Autodesk Inventor part; units mm, degrees
ref_plane "YZ Plane" through (0, 0, 0) normal (1, 0, 0) x (0, 1, 0)
ref_plane "XZ Plane" through (0, 0, 0) normal (0, 1, 0) x (-1, 0, 0)
ref_plane "XY Plane" through (0, 0, 0) normal (0, 0, 1) x (1, 0, 0)
sketch "スケッチ1" plane through (0, 0, 0) normal (0, 0, 1) x (1, 0, 0)
  line L0 (195, -7.5) -> (-195, -7.5)
  line L1 (-195, -7.5) -> (-195, 7.5)
  line L2 (-195, 7.5) -> (195, 7.5)
  line L3 (195, 7.5) -> (195, -7.5)
  line L4 (195, -7.5) -> (-195, 7.5) construction
  line L5 (-195, -7.5) -> (195, 7.5) construction
  circle A0 centre (0, 70.8153) radius 120
  line L6 (0, -7.5) -> (0, 7.5)
  circle A1 centre (-127.5, -22.5) radius 38
  line L7 (-175, -5) -> (-145, -5)
  line L8 (-145, -5) -> (-145, 5)
  line L9 (-145, 5) -> (-175, 5)
  line L10 (-175, 5) -> (-175, -5)
  line L11 (-195, 0) -> (195, 0)
  circle A2 centre (-175, 0) radius 1.6
  circle A3 centre (-165, 0) radius 1.6
  circle A4 centre (-155, 0) radius 1.6
  line L12 (0, 190.8153) -> (0, -49.1847)
  arc A5 (156.5411, -2.2739) -> (-157.0045, 0) centre (0, 30.8153) ccw
  arc A6 (161.433, -3.3079) -> (-162.968, 5) centre (0, 30.8153) ccw
  arc A7 (166.3249, -4.342) -> (-168.0285, 5) centre (0, 30.8153) ccw
  arc A8 (171.2168, -5.376) -> (-173.0854, 5) centre (0, 30.8153) ccw
  circle A9 centre (-169.2627, 15) radius 1.6
  circle A10 centre (-169.8998, 24.9797) radius 1.6
  line L13 (-164.9474, 34.9797) -> (-174.9504, 34.9797)
  line L14 (-175, -5) -> (-175, 30.8153)
  point P0 (0, 0)
  point P1 (-165, 0)
  point P2 (-175, 0)
  point P3 (-174.3906, 5)
  point P4 (-164.3536, 5)
  point P5 (-175, -1.6)
  point P6 (-175, 1.6)
  dimension "d0" = 390
  dimension "d1" = 15
  dimension "d2" = 240
  dimension "d3" = 76
  dimension "d4" = 30
  dimension "d5" = 67.5
  dimension "d9" = 10
  dimension "d10" = 10
  dimension "d11" = 20
  dimension "d13" = 10
  dimension "d14" = 10
  dimension "d16" = 3.2
  dimension "d17" = 3.2
  dimension "d19" = 3.2
  dimension "d28" = 40
  dimension "d29" = 5
  dimension "d30" = 5
  dimension "d31" = 5
  dimension "d32" = 3.2
  dimension "d33" = 3.2
  dimension "d34" = 15
  dimension "d35" = 10
  dimension "d36" = 10
extrude "押し出し1" add sketch "スケッチ1" along normal blind 3 contours L13 A7 A10 A9 L2 A8 | L11 A4 A5 A1 L9 L8 | L8 L7 A1 L11 A4 | L13 A6 L2 A7 A9 A10 | A8 L2 L14 | L7 L10 A2 L11 A3 A1 | A8 L9 L14 L2 | L2 A7 L9 A8 | L11 A3 A2 L10 L9 A5 A1 | A1 A5 L11 | A6 L9 A7 L2 | L9 A1 A5 | L10 L11 A2 | A2 L11 L10 picked at (-174.4361, -0.8975) picked at (-174.4361, 0.8975)
fillet "フィレット1" radius 5 6 edges at (-175, -5, 1.5) (-145, -5, 1.5) (-145, 5, 1.5) (-174.9504, 34.9797, 1.5) (-164.9474, 34.9797, 1.5) (-162.968, 5, 1.5)
properties part number "light_ball_space_nc"
Check sheet for the modelled part. Datum: model origin and axes. Units: mm. A direction names the side the tool comes from. Give positions to 0.01 mm unless a question says otherwise; leave off trailing zeros. Loops run counter-clockwise (first coordinate to the right, second up) from the corner with the lowest first, then second, coordinate; pieces in that order, holes last. Notation, with made-up numbers: M 44,43.5 L 57,43.5 A13 cw 57,52.5 Z; hole C 46.25,-0.5 d2. An arc over 180 degrees is marked long. Answer as a JSON object with one key per item and string values. Group by question number.
Q1. Cross-section at D-D on y = 18.5. Record the cut outline in (x, z).
Q2. Cross-section at A-A on x = -155. Record the cut outline in (y, z).
Q3. Material ranges on line 1 along X through (y, z) = (0, 1.8); line 2 along Y through (x, z) = (-155, 1.75); line 3 along Y through (x, z) = (-154.5, 0.6), recorded low to high. Write a range as [from, to].
Q4. Access from +Z, -Z, +X, -X, +Y, -Y to the whole of each face (thin tool, end or side, straight path). Record for faces 4 (the cylindrical face through (-147, -4, 2)), 5 (the flat face through (-154, 5, 1)).
Q5. Go/stop test with flat-tipped pins: P1, Ø0.9, axis at x = -154, z = 1.5, coming from the +Y side; P2, Ø3.5, axis at x = -169.26, y = 15, coming from the +Z side. Record where each tip stops, or that it passes through.
Q6. Release check for a two-part mould opening along Y. For faces 1 (the flat face through (-167, 11, 3)), 2 (the cylindrical face through (-163.52, 0.61, 1.48)), 3 (the cylindrical face through (-161.976, 6.275, 1.521)) record: released by +Y, released by -Y, zero draft, split by the parting line, or undercut.
Q7. Cross-section at B-B on y = 14.5. Record the cut outline in (x, z).
Q8. Cross-section at C-C on z = 1.4. Give the number of separate pieces and of enclosed holes in the cut face, then the cut area to 3 significant figures.
Evaluation:
{
 "1": {"outline": "M -175,0 L -164.54,0 L -164.54,3 L -175,3 Z"},
 "2": {"outline": "M -5,0 L -1.6,0 L -1.6,3 L -5,3 Z; M 1.6,0 L 5,0 L 5,3 L 1.6,3 Z"},
 "3": {"line 1": "x = [-175, -166.6], [-163.4, -156.6], [-153.4, -145]", "line 2": "y = [-5, -1.6], [1.6, 5]", "line 3": "y = [-5, -1.52], [1.52, 5]"},
 "4": {"face 4": "+Z, -Z, +X, -Y", "face 5": "+Z, -Z, +X, +Y"},
 "5": {"P1": "stops at y = 5", "P2": "stops at z = 3"},
 "6": {"face 1": "zero draft", "face 2": "undercut", "face 3": "released by +Y"},
 "7": {"outline": "M -175,0 L -170.78,0 L -170.78,3 L -175,3 Z; M -167.74,0 L -164.19,0 L -164.19,3 L -167.74,3 Z"},
 "8": {"separate pieces": "1", "enclosed holes": "4", "area": "562 mm2"}
}
